The figure shows three views and two pictorial views of one solid part (mm, origin at its lowest corner). Answer the questions. A direction names the side the tool comes from. Round coordinates to 2 decimals unless told otherwise and drop trailing zeros. Order: outer loops, then holes, each group sorted by start corner. A loop starts at its lowest first (then second) coordinate and runs counter-clockwise, first axis right, second up. Notation, with made-up numbers: (70, -24.75) -> (90, -24.75) arc R34 ccw to (90, 9.25) -> close; hole circle Ø8 at (79, 54). An arc over 180 degrees is marked (long way). Answer as a JSON object with one key per item and string values. Group by question number.
Item 1: Section B-B, the plane x = 194 is taken. Write down the section's boundary in (y, z), plus the area to 3 significant figures.
Item 2: The mould has two halves that part along Y. Classify the marked faces 4, 5 and 6: pulls with the +Y half, pulls with the -Y half, needs draft (parallel to the pull), parting line crosses it, or undercut.
Item 3: Section A-A, the plane z = 286 is taken. Write down the section's boundary in (x, y), plus the area to 3 significant figures.
Item 4: For the marked faces 1, 2 and 3, determine the directions among +Z, -Z, +X, -X, +Y, -Y from which every point of the face is accessible in a straight line to the end or side of a thin tool.
Item 5: Consider probe 1 along Y at (x, z) = (222.5, 186); probe 2 along Z at (x, y) = (275, 1144); probe 3 along Y at (x, z) = (164, 804). Determine where each line is inside the solid, lowest interval first. Write a range as from..to.
Item 6: Given P1, Ø12, axis at x = 227.5, y = 959, coming from the -Z side, flat-ended and moving along its own axis, determine where the tip first touches the part or whether it passes through.
Item 7: Section D-D, the plane y = 1606 is taken. Write down the section's boundary in (x, z).
Item 8: Section C-C, the plane y = 627 is taken. Write down the section's boundary in (x, z).
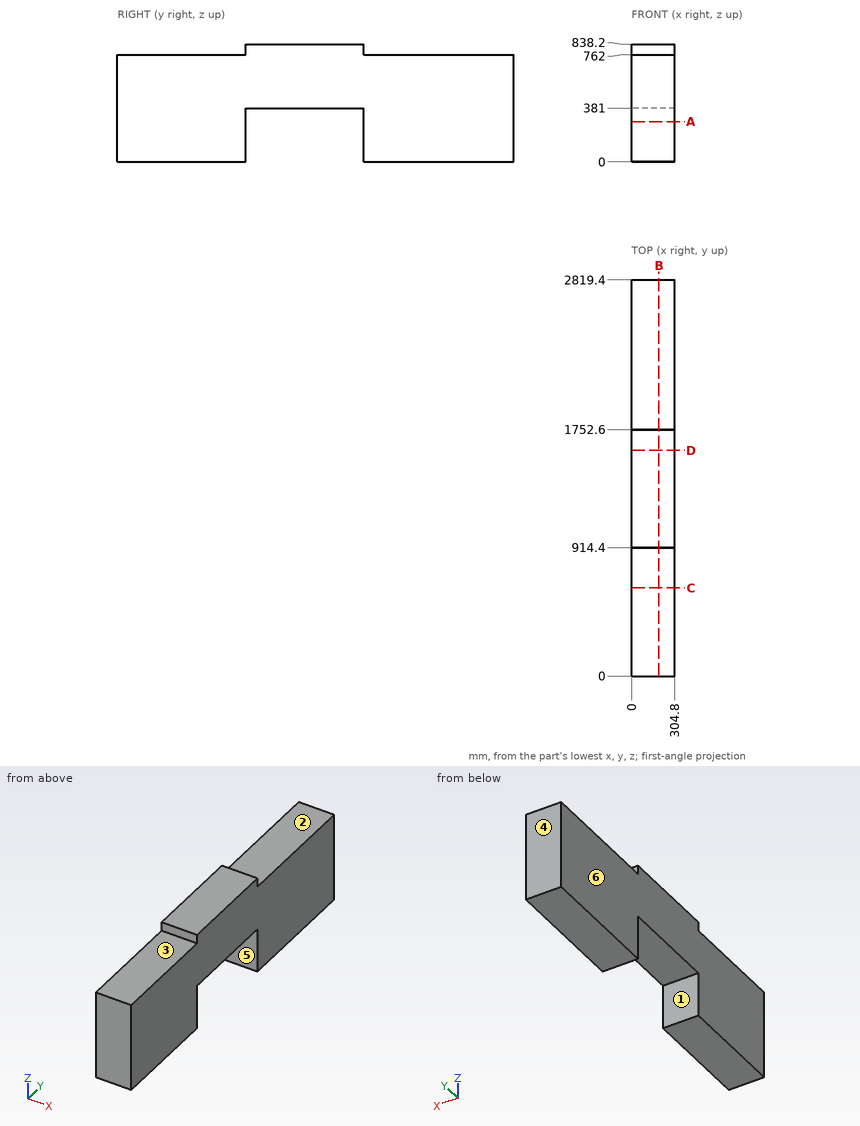
Values found:
{
 "1": {"outline": "(0, 0) -> (914.4, 0) -> (914.4, 381) -> (1752.6, 381) -> (1752.6, 0) -> (2819.4, 0) -> (2819.4, 762) -> (1752.6, 762) -> (1752.6, 838.2) -> (914.4, 838.2) -> (914.4, 762) -> (0, 762) -> close", "area": "1,890,000 mm2"},
 "2": {"face 4": "pulls with the +Y half", "face 5": "undercut", "face 6": "needs draft"},
 "3": {"outline": "(0, 0) -> (304.8, 0) -> (304.8, 914.4) -> (0, 914.4) -> close; (0, 1752.6) -> (304.8, 1752.6) -> (304.8, 2819.4) -> (0, 2819.4) -> close", "area": "604,000 mm2"},
 "4": {"face 1": "-Z, +X, -X", "face 2": "+Z, +X, -X, +Y", "face 3": "+Z, +X, -X, -Y"},
 "5": {"probe 1": "0..914.4, 1752.6..2819.4", "probe 2": "381..838.2", "probe 3": "914.4..1752.6"},
 "6": {"P1": "z = 381"},
 "7": {"outline": "(0, 381) -> (304.8, 381) -> (304.8, 838.2) -> (0, 838.2) -> close"},
 "8": {"outline": "(0, 0) -> (304.8, 0) -> (304.8, 762) -> (0, 762) -> close"}
}
